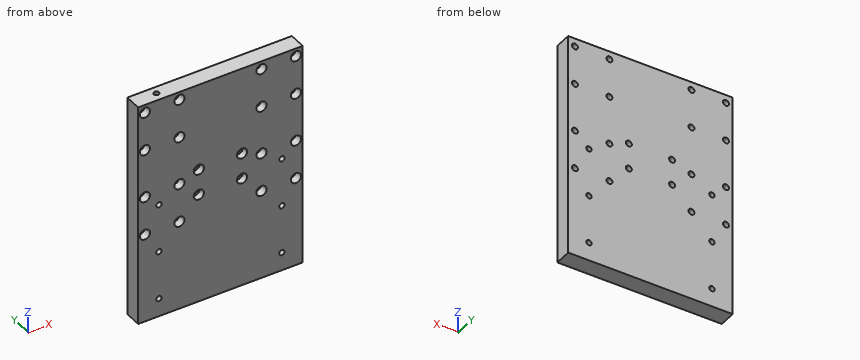
```python
from build123d import *

# Parameters (mm, degrees)
SKETCH003_W         = 152.5
SKETCH003_H         = 208
PAD001_DEPTH        = 7.85
HOLE_D              = 5.5
HOLE_CBORE_D        = 9.5
HOLE_CBORE_DEPTH    = 7.5
HOLE001_D           = 5.5
HOLE001_CBORE_D     = 9.5
HOLE001_CBORE_DEPTH = 6
SKETCH012_R         = 2.5
POCKET003_DEPTH     = 15.701
SKETCH016_R         = 2.5
POCKET006_DEPTH     = 25


with BuildPart() as part:
    # Sketch003 → Pad001 (new body, symmetric)
    with BuildSketch(Plane.XZ):
        with Locations((0, -38)):
            Rectangle(SKETCH003_W, SKETCH003_H)
    extrude(amount=PAD001_DEPTH, both=True)

    # Hole (through all)
    with Locations(Plane.XZ.offset(7.85)):
        with Locations((-70, 58.5), (-38, 58.5), (-70, 22.5), (-38, 22.5), (-70, -22.5), (-38, -22.5), (-70, -58.5), (-38, -58.5), (38, -22.5), (70, -22.5), (38, -58.5), (70, -58.5), (38, 22.5), (70, 22.5), (38, 58.5), (70, 58.5)):
            CounterBoreHole(HOLE_D / 2, HOLE_CBORE_D / 2, HOLE_CBORE_DEPTH)

    # Hole001 (through all)
    with Locations(Plane.XZ.offset(7.85)):
        with Locations((-20, -15.525), (20, -15.525), (-20, -39.525), (20, -39.525)):
            CounterBoreHole(HOLE001_D / 2, HOLE001_CBORE_D / 2, HOLE001_CBORE_DEPTH)

    # Sketch012 → Pocket003 (cut, through all)
    with BuildSketch(Plane.XZ.offset(7.85)):
        with Locations((-57, -80)):
            Circle(SKETCH012_R)
        with Locations((-57, -125)):
            Circle(SKETCH012_R)
        with Locations((57, -80)):
            Circle(SKETCH012_R)
        with Locations((57, -125)):
            Circle(SKETCH012_R)
        with Locations((-57, -35)):
            Circle(SKETCH012_R)
        with Locations((57, -35)):
            Circle(SKETCH012_R)
    extrude(amount=-POCKET003_DEPTH, mode=Mode.SUBTRACT)

    # Sketch016 (on Face1 of Pocket003) → Pocket006 (cut)
    with BuildSketch(Plane(origin=(0, 0, 66), x_dir=(-1, 0, 0), z_dir=(0, 0, 1))):
        with Locations((54, -0.4)):
            Circle(SKETCH016_R)
    extrude(amount=-POCKET006_DEPTH, mode=Mode.SUBTRACT)


with BuildPart() as part_1:
    # Body001 placement: moved
    add(part.part.moved(Location((88, -72, 0))))


solid = part_1.part
```
Geometry check sheet. Reference: the model listing, model coordinates, mm. Give positions to 0.01 mm unless a question says otherwise; leave off trailing zeros. Loops run counter-clockwise (first coordinate to the right, second up) from the corner with the lowest first, then second, coordinate; pieces in that order, holes last. Notation, with made-up numbers: M -20,35 L 17,35 A28 ccw 17,62 Z; hole C 4.25,-32 d3. An arc over 180 degrees is marked long. Write item = value, one per line. Start each with the question number.
1. Section check A-A, the plane x = 68. Enter the section's corners in (y, z) (3 decimals), plus the area to 3 significant figures.
2. Section check B-B, the plane x = 145. Enter the section's corners in (y, z), plus the area to 3 significant figures.
3. Thickness scan on probe 1 along Z at (x, y) = (126, -70); probe 2 along Z at (x, y) = (18, -76.5); probe 3 along X at (y, z) = (-74.5, -42.5). Record the ranges inside material, lowest first.
4. Section check C-C, the plane y = -77. Give the number of separate pieces and of enclosed holes in the cut face, plus the area to 3 significant figures.
5. Go/stop test with flat-tipped pins: P1, Ø4.5, axis at x = 34, y = -71.6, coming from the +Z side; P2, Ø5, axis at x = 68, z = -39.525, coming from the +Y side; P3, Ø7, axis at x = 50, z = -22.5, coming from the -Y side. Record where each tip stops, or that it passes through.
Values follow:
q1.outline = M -79.85,-142 L -64.15,-142 L -64.15,-42.275 L -73.85,-42.275 L -73.85,-44.275 L -79.85,-44.275 Z; M -79.85,-34.775 L -73.85,-34.775 L -73.85,-36.775 L -64.15,-36.775 L -64.15,-18.275 L -73.85,-18.275 L -73.85,-20.275 L -79.85,-20.275 Z; M -79.85,-10.775 L -73.85,-10.775 L -73.85,-12.775 L -64.15,-12.775 L -64.15,66 L -79.85,66 Z
q1.area = 3,040 mm^2
q2.outline = M -79.85,-142 L -64.15,-142 L -64.15,-127.5 L -79.85,-127.5 Z; M -79.85,-122.5 L -64.15,-122.5 L -64.15,-82.5 L -79.85,-82.5 Z; M -79.85,-77.5 L -64.15,-77.5 L -64.15,-37.5 L -79.85,-37.5 Z; M -79.85,-32.5 L -64.15,-32.5 L -64.15,66 L -79.85,66 Z
q2.area = 3,030 mm^2
q3.probe_1 = -142 to -61.25, -55.75 to -25.25, -19.75 to 19.75, 25.25 to 55.75, 61.25 to 66
q3.probe_2 = -142 to -63.25, -53.75 to -27.25, -17.75 to 17.75, 27.25 to 53.75, 63.25 to 66
q3.probe_3 = 11.75 to 64.3, 71.7 to 104.3, 111.7 to 164.25
q4.separate_pieces = 1
q4.enclosed_holes = 26
q4.area = 30,200 mm^2
q5.P1 = 41
q5.P2 = through
q5.P3 = -72.35
